Input: dimensioned drawing with shaded views. Units: mm. Origin: part minimum x, y, z. Give positions to 0.01 mm unless a question says otherwise; leave off trailing zeros. Write each loop counter-clockwise with the first axis right and the second up, starting at its lowest first coordinate (ties: lowest second). Pieces come first, ordered by that corner, then holes. Notation, with made-up numbers: (35, 87.25) -> (70, 87.25) arc R18 ccw to (70, 107.25) -> close; hole circle Ø4 at (7.5, 3). An arc over 180 degrees is marked (long way). Return JSON: item names as keys, results as strings. Group by question number.
Item 1: Pin query (flat end, axial travel): P1, Ø12, axis at x = 30, y = 25, coming from the +Z side. Return the tip coordinate at first contact, or that it passes through.
Item 2: Section A-A, the plane y = 33. Return loops of the section in (x, z).
Item 3: Section B-B, the plane x = 30. Return loops of the section in (y, z).
Item 4: Line query: line 1 (Y direction, x = 30, z = 18); line 2 (X direction, y = 28, z = 30.5); line 3 (X direction, y = 32.5, z = 17.5). Output: solid intervals per line, ascending. Write a range as [from, to].
Item 5: Mould query, pull axis X, two halves, no side actions, for the marked faces 1, 2 and 3. Classes: released by +X, released by -X, zero draft, split by the parting line, or undercut.
Item 6: Section C-C, the plane z = 28. Return loops of the section in (x, y).
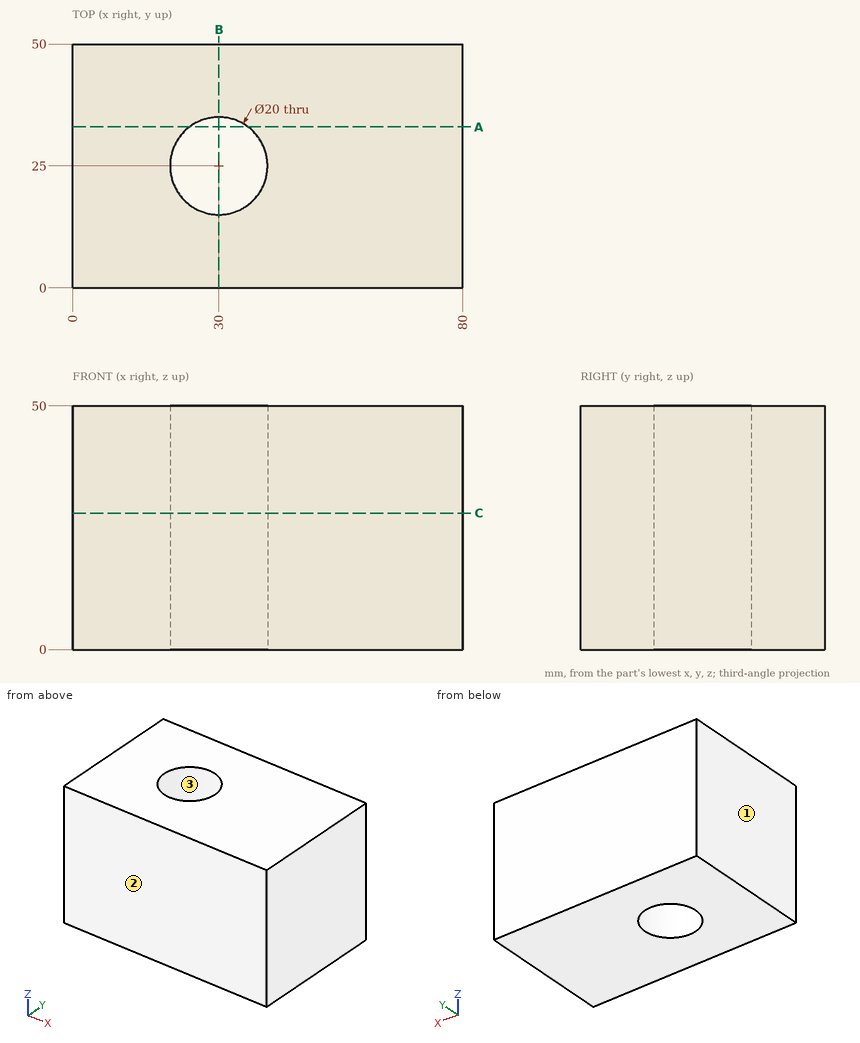
Answer below:
{
 "1": {"P1": "passes through"},
 "2": {"outline": "(0, 0) -> (24, 0) -> (24, 50) -> (0, 50) -> close; (36, 0) -> (80, 0) -> (80, 50) -> (36, 50) -> close"},
 "3": {"outline": "(0, 0) -> (15, 0) -> (15, 50) -> (0, 50) -> close; (35, 0) -> (50, 0) -> (50, 50) -> (35, 50) -> close"},
 "4": {"line 1": "y = [0, 15], [35, 50]", "line 2": "x = [0, 20.46], [39.54, 80]", "line 3": "x = [0, 23.39], [36.61, 80]"},
 "5": {"face 1": "released by -X", "face 2": "zero draft", "face 3": "undercut"},
 "6": {"outline": "(0, 0) -> (80, 0) -> (80, 50) -> (0, 50) -> close; hole circle Ø20 at (30, 25)"}
}
